Design review of the part built by this model. Coordinates are the model's own, in mm. Face numbers are marked on the shaded views. A direction names the side the tool comes from. Round coordinates to 2 decimals unless told otherwise and drop trailing zeros. Order: outer loops, then holes, each group sorted by start corner. A loop starts at its lowest first (then second) coordinate and runs counter-clockwise, first axis right, second up.
from build123d import *

# Parameters (mm, degrees)
SKETCH_1_W          = 6.5
SKETCH_1_H          = 6.9
EXTRUDE_1_DEPTH     = 3
EXTRUDE_START       = 3
SKETCH_1_3_R        = 3.25
EXTRUDE_2_DEPTH     = 1.7
CUT_EXTRUDE_START   = 3
CUT_EXTRUDE_1_DEPTH = 1.7
FILLET_1_R          = 2.5
SKETCH_2_W          = 1.8
SKETCH_2_H          = 3.4
EXTRUDE_3_DEPTH     = 0.3
SKETCH_3_W          = 2.3
SKETCH_3_H          = 0.3
EXTRUDE_4_DEPTH     = 1.9


with BuildPart() as part:
    # 草图1 → 凸台-拉伸1 (new body)
    with BuildSketch(Plane(origin=(0, 0, 0), x_dir=(1, 0, 0), z_dir=(0, 1, 0))):
        with Locations((0, -0.2)):
            Rectangle(SKETCH_1_W, SKETCH_1_H)
    extrude(amount=EXTRUDE_1_DEPTH)

    # 草图1<3> → 凸台-拉伸2 (add)
    with BuildSketch(Plane(origin=(0, 0, 0), x_dir=(1, 0, 0), z_dir=(0, 1, 0)).offset(EXTRUDE_START)):
        with Locations(Location((0, 0, 0), (0, 0, 90))):
            Circle(SKETCH_1_3_R)
        Polygon((-2.4, -0.5), (-2.4, 0.5), (-0.4, 0.5), (-0.4, 1.8), (0.4, 1.8), (0.4, 0.5), (2.4, 0.5), (2.4, -0.5), (0.4, -0.5), (0.4, -1.8), (-0.4, -1.8), (-0.4, -0.5), align=None, mode=Mode.SUBTRACT)
    extrude(amount=EXTRUDE_2_DEPTH)

    # 草图1<4> → 切除-拉伸1 (cut)
    with BuildSketch(Plane(origin=(0, 0, 0), x_dir=(1, 0, 0), z_dir=(0, 1, 0)).offset(CUT_EXTRUDE_START)):
        with BuildLine():
            Line((2.1914607, -2.4), (-2.1914607, -2.4))
            ThreePointArc((-2.1914607, -2.4), (0, -3.25), (2.1914607, -2.4))
        make_face()
    extrude(amount=CUT_EXTRUDE_1_DEPTH, mode=Mode.SUBTRACT)

    # 圆角1
    fillet_1_edges = [part.edges().sort_by_distance(p)[0] for p in [
        (-3.25, 1.5, -3.25),
        (3.25, 1.5, -3.25),
    ]]
    fillet(fillet_1_edges, radius=FILLET_1_R)

    # 草图2 → 凸台-拉伸3 (add)
    with BuildSketch(Plane.XY.offset(3.65)):
        with Locations((-2.25, -0.2)):
            Rectangle(SKETCH_2_W, SKETCH_2_H)
        with Locations((2.25, -0.2)):
            Rectangle(SKETCH_2_W, SKETCH_2_H)
    extrude(amount=EXTRUDE_3_DEPTH)

    # 草图3 → 凸台-拉伸4 (add)
    with BuildSketch(Plane.XZ):
        with Locations((0, -2.4)):
            Rectangle(SKETCH_3_W, SKETCH_3_H)
    extrude(amount=EXTRUDE_4_DEPTH)


solid = part.part
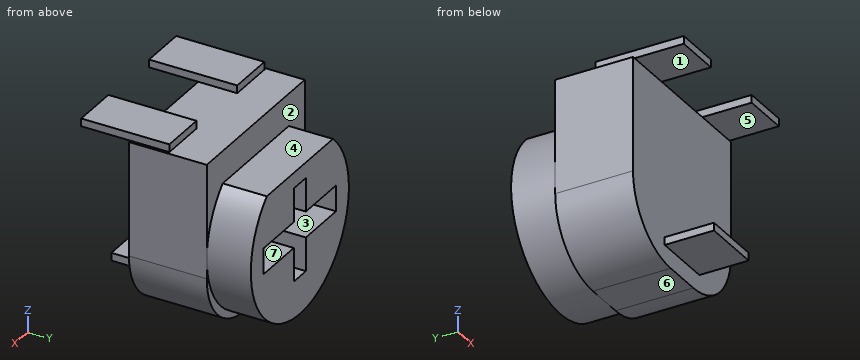
1) Take a section at C-C on y = 4.5. Give the boundary of the cut face in (x, z).
Results:
outline: (-2.19, 2.4) arc R3.25 ccw (long way) to (2.19, 2.4) - close; hole (-2.4, -0.5) - (-0.4, -0.5) - (-0.4, -1.8) - (0.4, -1.8) - (0.4, -0.5) - (2.4, -0.5) - (2.4, 0.5) - (0.4, 0.5) - (0.4, 1.8) - (-0.4, 1.8) - (-0.4, 0.5) - (-2.4, 0.5) - close
2) To check wall thickness, follow line 1 along Y through (x, z) = (1.5, -0.75); line 2 along Y through (x, z) = (-2.5, 3.25); line 3 along Z through (x, y) = (-0.75, 4.25). State the ranges of each line that lie inside material, in increasing order.
Results:
line 1: y = 0 to 4.7
line 2: y = 0 to 3
line 3: z = -3.16 to -0.5, 0.5 to 2.4
3) Take a section at D-D on z = 0.75. Give the boundary of the cut face in (x, y).
Results:
outline: (-3.25, 0) - (3.25, 0) - (3.25, 3) - (3.16, 3) - (3.16, 4.7) - (0.4, 4.7) - (0.4, 3) - (-0.4, 3) - (-0.4, 4.7) - (-3.16, 4.7) - (-3.16, 3) - (-3.25, 3) - close
4) Take a section at A-A on y = -1. Give the boundary of the cut face in (x, z).
Results:
outline: (-3.15, 3.65) - (-1.35, 3.65) - (-1.35, 3.95) - (-3.15, 3.95) - close; (-1.15, -2.55) - (1.15, -2.55) - (1.15, -2.25) - (-1.15, -2.25) - close; (1.35, 3.65) - (3.15, 3.65) - (3.15, 3.95) - (1.35, 3.95) - close
5) Take a section at B-B on y = 1. Give the boundary of the cut face in (x, z), plus the area to 3 significant figures.
Results:
outline: (-3.25, -0.75) arc R2.5 ccw to (-0.75, -3.25) - (0.75, -3.25) arc R2.5 ccw to (3.25, -0.75) - (3.25, 3.65) - (3.15, 3.65) - (3.15, 3.95) - (1.35, 3.95) - (1.35, 3.65) - (-1.35, 3.65) - (-1.35, 3.95) - (-3.15, 3.95) - (-3.15, 3.65) - (-3.25, 3.65) - close
area: 43.2 mm2
6) Clearance check with flat-ended pins moving along their axes: P1, Ø1.4, axis at x = -2, y = -1, coming from the -Z side; P2, Ø2, axis at x = -1.5, z = 0.5, coming from the -Y side; P3, Ø1.4, axis at y = 4, z = 1.5, coming from the +X side. State where each tip first meets the part, or that it passes through.
Results:
P1: stops at z = 3.65
P2: stops at y = 0
P3: stops at x = 3.15
7) The part is to be moulded in two halves that separate along Z. For the marked faces 1, 2, 3 and 4, say which applies: released by +Z, released by -Z, zero draft, split by the parting line, or undercut.
Results:
face 1: released by -Z
face 2: zero draft
face 3: undercut
face 4: released by +Z
8) For the marked faces 5, 6 and 7, list the 3-axis set-ups (+Z, -Z, +X, -X, +Y, -Y) from which the entire face can be reached by the end or side of a thin tool; tool diameter is ignored.
Results:
face 5: -Z, +X, -X, -Y
face 6: -Z, +X, -X, +Y, -Y
face 7: +Y
